```python
from build123d import *

# Parameters (mm, degrees)
ESQUISSE1_W             = 10
ESQUISSE1_H             = 5
BOSS_EXTRU_1_DEPTH      = 7.4
ESQUISSE2_W             = 6.6
ESQUISSE2_H             = 0.8
ENL_V_MAT_EXTRU_1_DEPTH = 8
ENL_V_MAT_EXTRU_2_DEPTH = 5.5
ESQUISSE5_W             = 6.8
ESQUISSE5_H             = 0.5
ESQUISSE5_W_2           = 0.5
ESQUISSE5_H_2           = 3.2
ENL_V_MAT_EXTRU_3_DEPTH = 1
ESQUISSE6_W             = 5.6
ESQUISSE6_H             = 0.5
ENL_V_MAT_EXTRU_4_DEPTH = 3
ESQUISSE8_W             = 6.6
ESQUISSE8_H             = 4.2
ENL_V_MAT_EXTRU_6_DEPTH = 1
BOSS_EXTRU_2_DEPTH      = 6.8
BOSS_EXTRU_3_DEPTH      = 2
BOSS_EXTRU_3_DEPTH_BACK = 2
ESQUISSE17_W            = 1.25
ESQUISSE17_H            = 4.2
BOSS_EXTRU_8_DEPTH      = 1
CHANFREIN1_SIZE         = 0.15
ESQUISSE13_W            = 0.45
ESQUISSE13_H            = 0.45
BOSS_EXTRU_5_DEPTH      = 0.8
BOSS_EXTRU_5_DEPTH_BACK = 6.3
CONG_2_R                = 0.1
ESQUISSE14_W            = 0.45
ESQUISSE14_H            = 0.43
BOSS_EXTRU_6_DEPTH      = 4.5
CHANFREIN2_SIZE         = 0.1
BOSS_EXTRU_7_DEPTH      = 7
CHANFREIN4_SIZE         = 0.15
CONG_3_R                = 0.1


with BuildPart() as part:
    # Esquisse1 → Boss.-Extru.1 (new body)
    with BuildSketch(Plane(origin=(0, 0, 0), x_dir=(1, 0, 0), z_dir=(0, 1, 0))):
        with Locations((5, 2.5)):
            Rectangle(ESQUISSE1_W, ESQUISSE1_H)
    extrude(amount=BOSS_EXTRU_1_DEPTH)

    # Esquisse2 → Enlèv. mat.-Extru.1 (cut)
    with BuildSketch(Plane(origin=(0, 7.4, 0), x_dir=(1, 0, 0), z_dir=(0, 1, 0))):
        with Locations((5, 0.4)):
            Rectangle(ESQUISSE2_W, ESQUISSE2_H)
    extrude(amount=-ENL_V_MAT_EXTRU_1_DEPTH, mode=Mode.SUBTRACT)

    # Esquisse4 → Enlèv. mat.-Extru.2 (cut)
    with BuildSketch(Plane(origin=(0, 7.4, 0), x_dir=(1, 0, 0), z_dir=(0, 1, 0))):
        Polygon((0.5, 0.5), (1.2, 0.5), (1.2, 1.3), (8.8, 1.3), (8.8, 0.5), (9.5, 0.5), (9.5, 4.5), (0.5, 4.5), align=None)
    extrude(amount=-ENL_V_MAT_EXTRU_2_DEPTH, mode=Mode.SUBTRACT)

    # Esquisse5 → Enlèv. mat.-Extru.3 (cut)
    with BuildSketch(Plane(origin=(0, 7.4, 0), x_dir=(1, 0, 0), z_dir=(0, 1, 0))):
        with Locations((5, 4.75)):
            Rectangle(ESQUISSE5_W, ESQUISSE5_H)
        with Locations((0.25, 2.9)):
            Rectangle(ESQUISSE5_W_2, ESQUISSE5_H_2)
        with Locations((9.75, 2.9)):
            Rectangle(ESQUISSE5_W_2, ESQUISSE5_H_2)
    extrude(amount=-ENL_V_MAT_EXTRU_3_DEPTH, mode=Mode.SUBTRACT)

    # Esquisse6 → Enlèv. mat.-Extru.4 (cut)
    with BuildSketch(Plane(origin=(0, 7.4, 0), x_dir=(1, 0, 0), z_dir=(0, 1, 0))):
        with Locations((5, 1.05)):
            Rectangle(ESQUISSE6_W, ESQUISSE6_H)
    extrude(amount=-ENL_V_MAT_EXTRU_4_DEPTH, mode=Mode.SUBTRACT)

    # Esquisse8 → Enlèv. mat.-Extru.6 (cut)
    with BuildSketch(Plane.XZ):
        with Locations((5, -2.9)):
            Rectangle(ESQUISSE8_W, ESQUISSE8_H)
    extrude(amount=-ENL_V_MAT_EXTRU_6_DEPTH, mode=Mode.SUBTRACT)

    # Esquisse9 → Boss.-Extru.2 (add)
    with BuildSketch(Plane(origin=(1.7, 0, 0), x_dir=(0, 0, -1), z_dir=(1, 0, 0))):
        Polygon((4.7, 1), (3.9, 0.2), (1.9, 0.2), (1.1, 1), align=None)
    extrude(amount=BOSS_EXTRU_2_DEPTH)

    # Esquisse11 → Boss.-Extru.3 (add, two sides)
    with BuildSketch(Plane(origin=(5, 0, 0), x_dir=(0, 0, -1), z_dir=(1, 0, 0))) as boss_extru_3_sk:
        Polygon((0.8, 4.4), (0.1, 2.8), (0.8, 2.8), align=None)
    extrude(amount=BOSS_EXTRU_3_DEPTH)
    extrude(boss_extru_3_sk.sketch, amount=-BOSS_EXTRU_3_DEPTH_BACK)

    # Esquisse17 → Boss.-Extru.8 (add)
    with BuildSketch(Plane(origin=(0, 1, 0), x_dir=(1, 0, 0), z_dir=(0, 1, 0))):
        with Locations((3.035, 2.9)):
            Rectangle(ESQUISSE17_W, ESQUISSE17_H)
        with Locations((5, 2.9)):
            Rectangle(ESQUISSE17_W, ESQUISSE17_H)
        with Locations((6.965, 2.9)):
            Rectangle(ESQUISSE17_W, ESQUISSE17_H)
    extrude(amount=-BOSS_EXTRU_8_DEPTH)

    # Chanfrein1
    chanfrein1_edges = [part.edges().sort_by_distance(p)[0] for p in [
        (2.2, 7.4, -1.05),
        (7.8, 7.4, -1.05),
    ]]
    chamfer(chanfrein1_edges, length=CHANFREIN1_SIZE)

    # Esquisse13 → Boss.-Extru.5 (add, two sides)
    with BuildSketch(Plane.XZ.offset(-0.2)) as boss_extru_5_sk:
        with Locations((8, -2.9)):
            Rectangle(ESQUISSE13_W, ESQUISSE13_H)
        with Locations((4, -2.9)):
            Rectangle(ESQUISSE13_W, ESQUISSE13_H)
        with Locations((2, -2.9)):
            Rectangle(ESQUISSE13_W, ESQUISSE13_H)
        with Locations((6, -2.9)):
            Rectangle(ESQUISSE13_W, ESQUISSE13_H)
    extrude(amount=BOSS_EXTRU_5_DEPTH)
    extrude(boss_extru_5_sk.sketch, amount=-BOSS_EXTRU_5_DEPTH_BACK)

    # Congé2
    cong_2_edges = [part.edges().sort_by_distance(p)[0] for p in [
        (0.25, 7.4, -1.3),
        (0, 7.4, -4.75),
        (1.6, 7.4, -4.75),
        (8.4, 7.4, -4.75),
        (10, 7.4, -4.75),
        (9.75, 7.4, -1.3),
    ]]
    fillet(cong_2_edges, radius=CONG_2_R)

    # Esquisse14 → Boss.-Extru.6 (add)
    with BuildSketch(Plane(origin=(0, 0, -3.125), x_dir=(-1, 0, 0), z_dir=(0, 0, -1))):
        with Locations((-8, -0.385)):
            Rectangle(ESQUISSE14_W, ESQUISSE14_H)
        with Locations((-6, -0.385)):
            Rectangle(ESQUISSE14_W, ESQUISSE14_H)
        with Locations((-4, -0.385)):
            Rectangle(ESQUISSE14_W, ESQUISSE14_H)
        with Locations((-2, -0.385)):
            Rectangle(ESQUISSE14_W, ESQUISSE14_H)
    extrude(amount=-BOSS_EXTRU_6_DEPTH)

    # Chanfrein2
    chanfrein2_edges = [part.edges().sort_by_distance(p)[0] for p in [
        (4.225, 6.5, -2.9),
        (4, 6.5, -3.125),
        (3.775, 6.5, -2.9),
        (4, 6.5, -2.675),
        (2.225, 6.5, -2.9),
        (2, 6.5, -3.125),
        (1.775, 6.5, -2.9),
        (2, 6.5, -2.675),
        (8, 6.5, -3.125),
        (7.775, 6.5, -2.9),
        (8, 6.5, -2.675),
        (8.225, 6.5, -2.9),
        (6, 6.5, -3.125),
        (5.775, 6.5, -2.9),
        (6, 6.5, -2.675),
        (6.225, 6.5, -2.9),
        (8.225, -0.385, 1.375),
        (8, -0.17, 1.375),
        (7.775, -0.385, 1.375),
        (8, -0.6, 1.375),
        (6.225, -0.385, 1.375),
        (6, -0.17, 1.375),
        (5.775, -0.385, 1.375),
        (6, -0.6, 1.375),
        (4.225, -0.385, 1.375),
        (4, -0.17, 1.375),
        (3.775, -0.385, 1.375),
        (4, -0.6, 1.375),
        (2.225, -0.385, 1.375),
        (2, -0.17, 1.375),
        (1.775, -0.385, 1.375),
        (2, -0.6, 1.375),
    ]]
    chamfer(chanfrein2_edges, length=CHANFREIN2_SIZE)

    # Esquisse16 → Boss.-Extru.7 (add)
    with BuildSketch(Plane(origin=(0, 6.4, 0), x_dir=(1, 0, 0), z_dir=(0, 1, 0))):
        Polygon((0, 1.3), (-0.2, 1.3), (-0.2, 1.8), (-1, 1.8), (-1, 1.3), (-1, 0), (0, 0), align=None)
        Polygon((-0.2, 4.5), (-0.2, 3.9), (-1, 3.9), (-1, 5), (-0.2, 5), (0, 5), (0, 4.5), align=None)
        Polygon((11, 3.9), (10.2, 3.9), (10.2, 4.5), (10, 4.5), (10, 5), (10.2, 5), (11, 5), align=None)
        Polygon((11, 1.3), (11, 1.8), (10.2, 1.8), (10.2, 1.3), (10, 1.3), (10, 0), (11, 0), align=None)
    extrude(amount=-BOSS_EXTRU_7_DEPTH)

    # Chanfrein4
    chanfrein4_edges = [part.edges().sort_by_distance(p)[0] for p in [
        (-0.6, 6.4, -1.8),
        (-0.6, 6.4, -3.9),
        (10.6, 6.4, -3.9),
        (10.6, 6.4, -1.8),
    ]]
    chamfer(chanfrein4_edges, length=CHANFREIN4_SIZE)

    # Congé3
    cong_3_edges = [part.edges().sort_by_distance(p)[0] for p in [
        (4, -0.6, -3.125),
        (2, -0.6, -3.125),
        (8, -0.6, -3.125),
        (6, -0.6, -3.125),
        (8, -0.17, -2.675),
        (6, -0.17, -2.675),
        (4, -0.17, -2.675),
        (2, -0.17, -2.675),
    ]]
    fillet(cong_3_edges, radius=CONG_3_R)


solid = part.part
```
Geometry check sheet. Reference: the model listing, model coordinates, mm. A direction names the side the tool comes from. Give positions to 0.01 mm unless a question says otherwise; leave off trailing zeros. Order: outer loops, then holes, each group sorted by start corner. A loop starts at its lowest first (then second) coordinate and runs counter-clockwise, first axis right, second up.
1. Release check for a two-part mould opening along X. For faces 5 (the face through (-0.5, -0.6, -4.5)), 6 (the face through (5, 0, -3)), 7 (the face through (0, 7, -1)), 8 (the face through (0.5, 4, -3)) record: pulls with the +X half, pulls with the -X half, needs draft (parallel to the pull), parting line crosses it, or undercut.
2. Section check A-A, the plane z = 0.5. Enter the section's corners in (x, y) (3 decimals).
3. Section check B-B, the plane y = 2.25. Give the number of separate pieces and of enclosed holes in the cut face, and give its area (3 significant figures).
4. Access from +Z, -Z, +X, -X, +Y, -Y to the whole of each face (thin tool, end or side, straight path). Record for faces 1 (the face through (-0.5, 6.4, -4.5)), 2 (the face through (1, 0, -3)), 3 (the face through (0, 3, -3)), 4 (the face through (7.9, 0.6, -4.3)).
5. Gauge pin test, flat ends, axial feed: pin 1 Ø3 at (x, y) = (1.5, 2.5) entering from +Z; pin 2 Ø0.5 at (x, z) = (9, -2.5) entering from -Y; pin 3 Ø0.5 at (y, z) = (5, -3) entering from +X. Record the tip position at first contact, or that the pin passes through.
6. Section check C-C, the plane x = 7.25. Enter the section's corners in (y, z), and give its area (3 significant figures).
7. Thickness scan on L1, parallel to X at y = 2, z = -2.75 (3 decimals); L2, parallel to X at y = 3.5, z = -0.75; L3, parallel to X at y = 1.5, z = -0.5. Record the ranges inside material, lowest first.
Values follow:
1. face 5: needs draft
1. face 6: undercut
1. face 7: pulls with the -X half
1. face 8: undercut
2. outline: (1.775, -0.6) - (2.225, -0.6) - (2.225, -0.17) - (1.775, -0.17) - close; (3.775, -0.6) - (4.225, -0.6) - (4.225, -0.17) - (3.775, -0.17) - close; (5.775, -0.6) - (6.225, -0.6) - (6.225, -0.17) - (5.775, -0.17) - close; (7.775, -0.6) - (8.225, -0.6) - (8.225, -0.17) - (7.775, -0.17) - close
3. separate pieces: 5
3. enclosed holes: 1
3. area: 21.0 mm2
4. face 1: +Z, -Z, -X, +Y
4. face 2: +Z, -Z, -Y
4. face 3: +Y, -Y
4. face 4: -Z, -Y
5. pin 1: stops at z = 0
5. pin 2: stops at y = 0
5. pin 3: stops at x = 10
6. outline: (0, -5) - (6.4, -5) - (6.4, -4.5) - (1.9, -4.5) - (1.9, -1.3) - (4.4, -1.3) - (4.4, -0.8) - (0, -0.8) - close
6. area: 11.5 mm2
7. L1: x = 0 to 0.5, 1.775 to 2.225, 3.775 to 4.225, 5.775 to 6.225, 7.775 to 8.225, 9.5 to 10
7. L2: x = -1 to 0.5, 1.2 to 1.7, 3 to 7, 8.3 to 8.8, 9.5 to 11
7. L3: x = -1 to 1.7, 8.3 to 11
